Geometry: see drawing. Coordinates: mm, zero at the bounding-box minimum. Give positions to 0.01 mm unless a question says otherwise; leave off trailing zeros. Loops run counter-clockwise (first coordinate to the right, second up) from the corner with the lowest first, then second, coordinate; pieces in that order, holes last. Notation, with made-up numbers: (10.25, 80.25) -> (69.25, 80.25) arc R26 cw to (69.25, 107.25) -> close; hole circle Ø5 at (71, 36). An arc over 180 degrees is marked (long way). Return JSON: item names as keys, results as strings. Group by question number.
(1) Cut plane C-C on y = 10.75. Return loops of the section in (x, z).
(2) Cut plane D-D on z = 90. Return loops of the section in (x, y), then the cut area to 3 significant figures.
(3) Draft query along X for the marked faces 1, 2 and 3. Return one class per face: released by +X, released by -X, zero draft, split by the parting line, or undercut.
(4) Cut plane A-A on x = 80. Return loops of the section in (y, z), then the cut area to 3 significant figures.
(5) Cut plane B-B on z = 49.5. Return loops of the section in (x, y), then the cut area to 3 significant figures.
(6) Pin query (flat end, axial travel): pin 1 (5 mm diameter, centred on y = 12, z = 41.5, fed in from -X); pin 2 (4 mm diameter, centred on x = 86, y = 4.5, fed in from -Z). Return the tip coordinate at first contact, or that it passes through.
(7) Ray query, line 1 (X direction, y = 4.75, z = 89); line 2 (Z direction, x = 145, y = 11.25); line 3 (Z direction, x = 80, y = 3.25). Return the intervals inside material, ascending. Write a range as from..to.
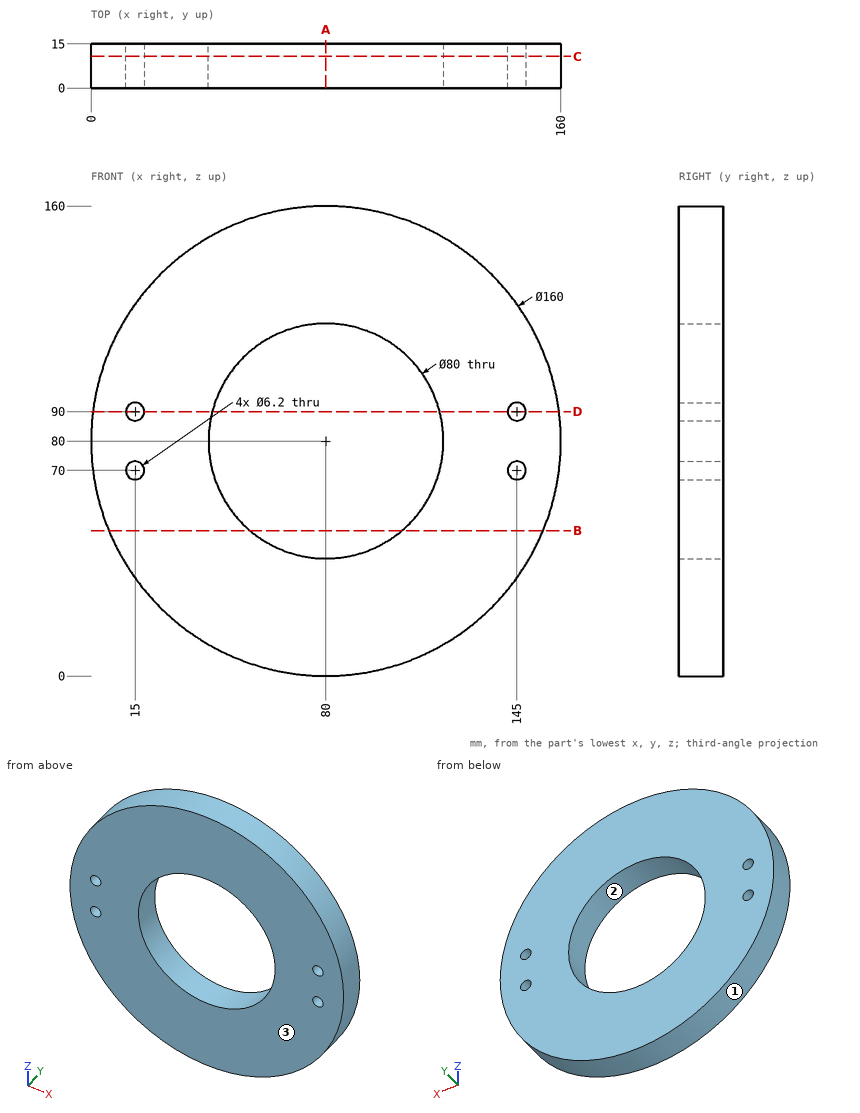
Answers:
{
 "1": {"outline": "circle Ø160 at (80, 80); hole circle Ø6.2 at (15, 70); hole circle Ø6.2 at (15, 90); hole circle Ø80 at (80, 80); hole circle Ø6.2 at (145, 70); hole circle Ø6.2 at (145, 90)"},
 "2": {"outline": "(0.63, 0) -> (11.9, 0) -> (11.9, 15) -> (0.63, 15) -> close; (18.1, 0) -> (41.27, 0) -> (41.27, 15) -> (18.1, 15) -> close; (118.73, 0) -> (141.9, 0) -> (141.9, 15) -> (118.73, 15) -> close; (148.1, 0) -> (159.37, 0) -> (159.37, 15) -> (148.1, 15) -> close", "area": "1,030 mm²"},
 "3": {"face 1": "split by the parting line", "face 2": "undercut", "face 3": "zero draft"},
 "4": {"outline": "(0, 0) -> (15, 0) -> (15, 40) -> (0, 40) -> close; (0, 120) -> (15, 120) -> (15, 160) -> (0, 160) -> close", "area": "1,200 mm²"},
 "5": {"outline": "(6.04, 0) -> (54.12, 0) -> (54.12, 15) -> (6.04, 15) -> close; (105.88, 0) -> (153.96, 0) -> (153.96, 15) -> (105.88, 15) -> close", "area": "1,440 mm²"},
 "6": {"pin 1": "x = 8.56", "pin 2": "z = 0.1"},
 "7": {"line 1": "0.51..12.07, 17.93..41.03, 118.97..142.07, 147.93..159.49", "line 2": "33.36..66.9, 73.1..86.9, 93.1..126.64", "line 3": "0..40, 120..160"}
}
